Can you work these out from the model? Positions are in its coordinate system, mm. Face numbers are marked on the shaded views. A direction names the side the tool comes from. Coordinates: 2 decimals unless noted, no trailing zeros. Order: outer loops, then holes, each group sorted by start corner. A loop starts at its lowest first (then second) coordinate and runs counter-clockwise, first axis right, second up. Notation, with made-up numbers: (-20.75, 53) -> (-0.75, 53) arc R20 cw to (-0.75, 66) -> close; hole circle Ø5 at (83, 2.5). An arc over 180 degrees is marked (long way). Answer in a Markdown table with one row per item. Add a question column.
1. Will these pins go through, and if not, where does the flat tip stop? pin 1 (10 mm diameter, centred on x = -381, y = 197, fed in from +Z); pin 2 (19.5 mm diameter, centred on x = -263.5, y = 57, fed in from +Z).
2. Imagine slicing it at B-B on z = 116. Write out the boundary of the cut face in (x, y).
3. If I drill on line 1 along Y through (x, z) = (-16, -3); line 2 along X through (y, z) = (16.5, 207.5); line 3 along Y through (x, z) = (-79, 111), over which ranges is the centre line in solid material (lowest first)? Write a range as [from, to].
4. On a 3-axis mill with a long thin cutter (end or side, diameter ignored), from which of +Z, -Z, +X, -X, +Y, -Y can I reach the whole of each face in a straight line? I mean the marked faces 1, 2 and 3. Say none if no direction works.
5. Imagine slicing it at C-C on x = -97. Write out the boundary of the cut face in (y, z), plus the area to 3 significant figures.
6. We'd pull the mould along X, two halves only. Please class the marked faces 4, 5, 6 and 7: pulls with the +X half, pulls with the -X half, needs draft (parallel to the pull), parting line crosses it, or undercut.
7. Imagine slicing it at D-D on y = 92. Write out the boundary of the cut face in (x, z).
8. Imagine slicing it at A-A on z = 33. Write out the boundary of the cut face in (x, y), plus the area to 3 significant figures.
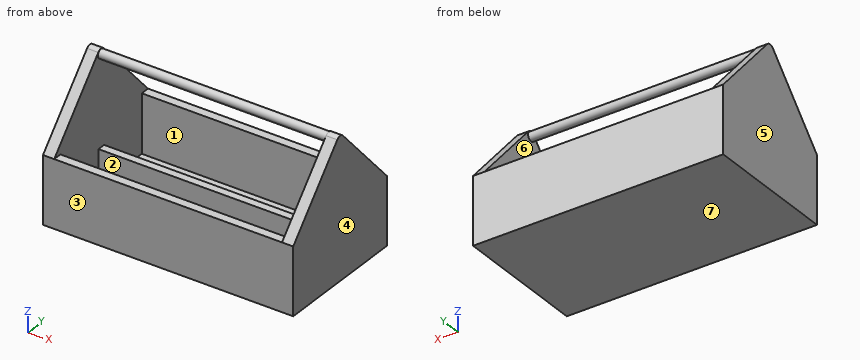
from build123d import *

# Parameters (mm, degrees)
F1_DEPTH = 25
F3_DEPTH = 508
F5_DEPTH = 25
F6_R     = 10
F7_DEPTH = 508
F8_W     = 508
F8_H     = 17.884616
F9_DEPTH = 80


with BuildPart() as f1:
    # F0 (on Right) → F1 (new body)
    with BuildSketch(Plane.YZ):
        with BuildLine():
            Line((-97.451926, 123.666471), (-97.451926, -26.333529))
            Line((-97.451926, -26.333529), (202.548074, -26.333529))
            Line((202.548074, -26.333529), (202.548074, 123.666471))
            Line((202.548074, 123.666471), (61.499769, 281.658165))
            ThreePointArc((61.499769, 281.658165), (52.548074, 285.666471), (43.59638, 281.658165))
            Line((43.59638, 281.658165), (-97.451926, 123.666471))
        make_face()
    extrude(amount=F1_DEPTH)

    # F2 (on face) → F3 (join)
    with BuildSketch(Plane(origin=(0, 0, 0), x_dir=(0, -1, 0), z_dir=(-1, 0, 0))):
        Polygon((-182.548074, 123.666471), (-202.548074, 123.666471), (-202.548074, -26.333529), (97.451926, -26.333529), (97.451926, 123.666471), (77.451926, 123.666471), (77.451926, -6.333529), (-182.548074, -6.333529), align=None)
    extrude(amount=F3_DEPTH)

    # F4 (on face) → F5 (join)
    with BuildSketch(Plane(origin=(-508, 0, 0), x_dir=(0, -1, 0), z_dir=(-1, 0, 0))):
        with BuildLine():
            Line((97.451926, 123.666471), (-43.59638, 281.658165))
            ThreePointArc((-43.59638, 281.658165), (-52.548074, 285.666471), (-61.499769, 281.658165))
            Line((-61.499769, 281.658165), (-202.548074, 123.666471))
            Line((-202.548074, 123.666471), (-202.548074, -26.333529))
            Line((-202.548074, -26.333529), (97.451926, -26.333529))
            Line((97.451926, -26.333529), (97.451926, 123.666471))
        make_face()
    extrude(amount=F5_DEPTH)

    # F6 (on face) → F7 (join)
    with BuildSketch(Plane.YZ):
        with Locations((52.24314, 274.906725)):
            Circle(F6_R)
    extrude(amount=-F7_DEPTH)

    # F8 (on face) → F9 (join)
    with BuildSketch(Plane.XY.offset(-6.333529)):
        with Locations((-254, 53.124996)):
            Rectangle(F8_W, F8_H)
    extrude(amount=F9_DEPTH)


solid = f1.part
Answers follow:
| question | item | result |
|---|---|---|
| 1 | pin 1 | stops at z = 123.67 |
| 1 | pin 2 | stops at z = 284.91 |
| 2 | outline | (-533, -97.45) -> (25, -97.45) -> (25, 202.55) -> (-533, 202.55) -> close; hole (-508, -77.45) -> (0, -77.45) -> (0, 182.55) -> (-508, 182.55) -> close |
| 3 | line 1 | y = [-97.45, -77.45], [44.18, 62.07], [182.55, 202.55] |
| 3 | line 2 | x = [-533, -508], [0, 25] |
| 3 | line 3 | y = [-97.45, -77.45], [182.55, 202.55] |
| 4 | face 1 | +Z |
| 4 | face 2 | none |
| 4 | face 3 | +Z, -Z, +X, -X, -Y |
| 5 | outline | (-97.45, -26.33) -> (202.55, -26.33) -> (202.55, 123.67) -> (182.55, 123.67) -> (182.55, -6.33) -> (62.07, -6.33) -> (62.07, 73.67) -> (44.18, 73.67) -> (44.18, -6.33) -> (-77.45, -6.33) -> (-77.45, 123.67) -> (-97.45, 123.67) -> close; circle Ø20 at (52.24, 274.91) |
| 5 | area | 12,900 mm² |
| 6 | face 4 | pulls with the +X half |
| 6 | face 5 | pulls with the -X half |
| 6 | face 6 | undercut |
| 6 | face 7 | needs draft |
| 7 | outline | (-533, -26.33) -> (25, -26.33) -> (25, 247.49) -> (0, 247.49) -> (0, -6.33) -> (-508, -6.33) -> (-508, 247.49) -> (-533, 247.49) -> close |
| 8 | outline | (-533, -97.45) -> (25, -97.45) -> (25, 202.55) -> (-533, 202.55) -> close; hole (-508, -77.45) -> (0, -77.45) -> (0, 44.18) -> (-508, 44.18) -> close; hole (-508, 62.07) -> (0, 62.07) -> (0, 182.55) -> (-508, 182.55) -> close |
| 8 | area | 44,400 mm² |
